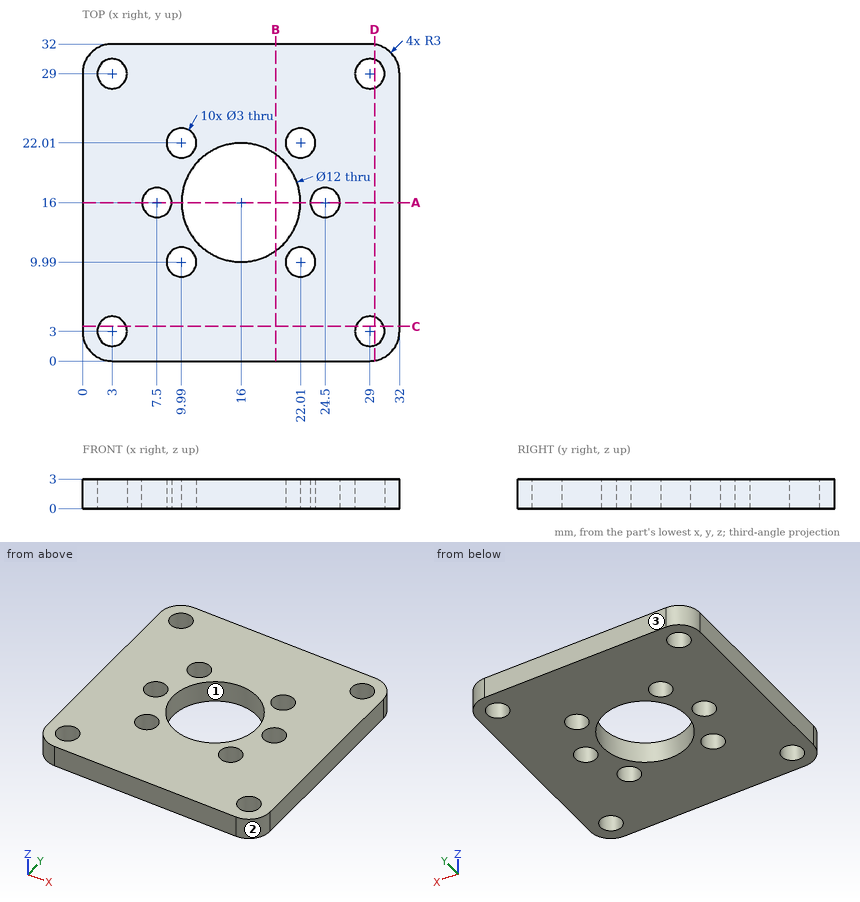
For this review, use the dimensioned drawing (mm, ordinates from the lowest corner) and the shaded views. Give positions to 0.01 mm unless a question says otherwise; leave off trailing zeros. Order: outer loops, then holes, each group sorted by start corner. A loop starts at its lowest first (then second) coordinate and runs counter-clockwise, first axis right, second up.
1. Add section A-A, the plane y = 16. State the section outline as (x, z) points, then the cut area to 3 significant figures.
Solution:
outline: (0, 0) - (6, 0) - (6, 3) - (0, 3) - close; (9, 0) - (10, 0) - (10, 3) - (9, 3) - close; (22, 0) - (23, 0) - (23, 3) - (22, 3) - close; (26, 0) - (32, 0) - (32, 3) - (26, 3) - close
area: 42.0 mm2
2. Mouldability with a two-part tool opening along X and no side actions: class the marked faces 1, 2 and 3 as +X half, -X half, draft (parallel to the pull), parting line (faces both ways), or undercut.
Solution:
face 1: undercut
face 2: +X half
face 3: draft
3. To check wall thickness, follow L1, parallel to Y at x = 7.5, z = 1.05; L2, parallel to X at y = 16.5, z = 2.6 (1 decimal); L3, parallel to Y at x = 10.5, z = 1.5 (1 decimal). State the ranges of each line that lie inside material, in increasing order.
Solution:
L1: y = 0 to 14.5, 17.5 to 32
L2: x = 0 to 6.1, 8.9 to 10, 22 to 23.1, 25.9 to 32
L3: y = 0 to 8.6, 11.4 to 13.6, 18.4 to 20.6, 23.4 to 32
4. Add section B-B, the plane x = 19.5. State the section outline as (y, z) points.
Solution:
outline: (0, 0) - (11.13, 0) - (11.13, 3) - (0, 3) - close; (20.87, 0) - (32, 0) - (32, 3) - (20.87, 3) - close
5. Add section C-C, the plane y = 3.5. State the section outline as (x, z) points (1 decimal).
Solution:
outline: (0, 0) - (1.6, 0) - (1.6, 3) - (0, 3) - close; (4.4, 0) - (27.6, 0) - (27.6, 3) - (4.4, 3) - close; (30.4, 0) - (32, 0) - (32, 3) - (30.4, 3) - close
6. For pin 1 Ø15.5 at (x, y) = (16, 16) entering from +Z, flat-tipped, find the tip position at first contact; note if it passes through.
Solution:
pin 1: stops at z = 3
